```python
from build123d import *

# Parameters (mm, degrees)
SKETCH2_R           = 30
BOSS_EXTRUDE1_DEPTH = 80
SKETCH3_R           = 26.016919331
CUT_EXTRUDE4_DEPTH  = 75
SKETCH5_W           = 40
SKETCH5_H           = 10
CUT_EXTRUDE6_DEPTH  = 91.553851381
SKETCH6_R           = 1.983080669
BOSS_EXTRUDE2_DEPTH = 63


with BuildPart() as part:
    # Sketch2 → Boss-Extrude1 (new body)
    with BuildSketch(Plane(origin=(0, 0, 0), x_dir=(1, 0, 0), z_dir=(0, 1, 0))):
        with Locations(Location((0, 0, 0), (0, 0, 270))):
            Circle(SKETCH2_R)
    extrude(amount=BOSS_EXTRUDE1_DEPTH)

    # Sketch3 → Cut-Extrude4 (cut)
    with BuildSketch(Plane(origin=(0, 80, 0), x_dir=(1, 0, 0), z_dir=(0, 1, 0))):
        with Locations(Location((0, 0, 0), (0, 0, 270))):
            Circle(SKETCH3_R)
    extrude(amount=-CUT_EXTRUDE4_DEPTH, mode=Mode.SUBTRACT)

    # Sketch5 → Cut-Extrude6 (cut, through all)
    with BuildSketch(Plane(origin=(0, 0, 0), x_dir=(0, 0, -1), z_dir=(1, 0, 0))):
        with Locations((0, 6.124342534)):
            Rectangle(SKETCH5_W, SKETCH5_H)
    extrude(amount=-CUT_EXTRUDE6_DEPTH, mode=Mode.SUBTRACT)

    # Sketch6 → Boss-Extrude2 (add)
    with BuildSketch(Plane(origin=(0, 80, 0), x_dir=(1, 0, 0), z_dir=(0, 1, 0))):
        with Locations((26.016919331, 0)):
            Circle(SKETCH6_R)
        with Locations((-26.016919331, 0)):
            Circle(SKETCH6_R)
        with Locations((0, -26.016919331)):
            Circle(SKETCH6_R)
        with Locations((0, 26.016919331)):
            Circle(SKETCH6_R)
    extrude(amount=-BOSS_EXTRUDE2_DEPTH)


solid = part.part
```
Design review of the part built by this model. Coordinates are the model's own, in mm. A direction names the side the tool comes from. Coordinates: 2 decimals unless noted, no trailing zeros. Order: outer loops, then holes, each group sorted by start corner. A loop starts at its lowest first (then second) coordinate and runs counter-clockwise, first axis right, second up.
1) Take a section at A-A, the plane y = 66.5. Give the boundary of the cut face in (x, z).
2) Mouldability with a two-part tool opening along Z and no side actions: class faces 5 (the cylindrical face through (29.745, 39.44, -3.905)), 6 (the cylindrical face through (-24.034, 48.941, 0.043)), 7 (the flat face through (25, 80, 0)), 8 (the flat face through (10, 5, 0)) as +Z half, -Z half, draft (parallel to the pull), parting line (faces both ways), or undercut.
3) Take a section at B-B, the plane z = -5. Give the boundary of the cut face in (x, y), and give its area (3 significant figures).
4) Take a section at D-D, the plane z = 8. Give the boundary of the cut face in (x, y), and give its area (3 significant figures).
5) Take a section at C-C, the plane x = 17. Give the boundary of the cut face in (y, z).
6) For faces 1 (the flat face through (0, 0, 0)), 2 (the flat face through (0, 3, 0)), 3 (the flat face through (-25, 17, 0)), 4 (the flat face through (-14, 4, 20)), list the 3-axis set-ups (+Z, -Z, +X, -X, +Y, -Y) from which the entire face can be reached by the end or side of a thin tool; tool diameter is ignored.
7) Clearance check with flat-ended pins moving along their axes: pin 1 (3 mm diameter, centred on y = 3, z = -1, fed in from -X); pin 2 (12 mm diameter, centred on x = 22, y = 19.5, fed in from -Z); pin 3 (3 mm diameter, centred on x = 11, y = 36.5, fed in from +Z). State where each tip first meets the part, or that it passes through.
8) Wall thickness on line 1 along X through (y, z) = (30, 0); line 2 along Y through (x, z) = (-23, -18); line 3 along Y through (x, z) = (5, 21): over which ranges is each line inside the solid? List them lowest first.
Returned:
1. outline: circle Ø60 at (0, 0); hole (-25.94, -1.98) arc R26.02 ccw to (-1.98, -25.94) arc R1.98 cw to (1.98, -25.94) arc R26.02 ccw to (25.94, -1.98) arc R1.98 cw to (25.94, 1.98) arc R26.02 ccw to (1.98, 25.94) arc R1.98 cw to (-1.98, 25.94) arc R26.02 ccw to (-25.94, 1.98) arc R1.98 cw to start
2. face 5: parting line
2. face 6: undercut
2. face 7: draft
2. face 8: undercut
3. outline: (-29.58, 0) - (29.58, 0) - (29.58, 80) - (25.53, 80) - (25.53, 5) - (0, 5) - (0, 1.12) - (-29.58, 1.12) - close; (-29.58, 11.12) - (-25.53, 11.12) - (-25.53, 80) - (-29.58, 80) - close
3. area: 764 mm2
4. outline: (-28.91, 0) - (28.91, 0) - (28.91, 80) - (24.76, 80) - (24.76, 5) - (0, 5) - (0, 1.12) - (-28.91, 1.12) - close; (-28.91, 11.12) - (-24.76, 11.12) - (-24.76, 80) - (-28.91, 80) - close
4. area: 775 mm2
5. outline: (0, -24.72) - (80, -24.72) - (80, -19.69) - (5, -19.69) - (5, 19.69) - (80, 19.69) - (80, 24.72) - (0, 24.72) - close
6. face 1: +Z, -Z, +X, -X, -Y
6. face 2: -X, +Y
6. face 3: none
6. face 4: -X
7. pin 1: stops at x = 0
7. pin 2: stops at z = -25.38
7. pin 3: stops at z = 28.46
8. line 1: x = -30 to -24.03, 24.03 to 30
8. line 2: y = 0 to 1.12, 11.12 to 80
8. line 3: y = 0 to 5
